Verification items for the finished model (mm, model axes). Face numbers are marked on the shaded views. Give positions to 0.01 mm unless a question says otherwise; leave off trailing zeros. Write each loop counter-clockwise with the first axis right and the second up, starting at its lowest first coordinate (ties: lowest second). Pieces come first, ordered by that corner, then holes. Notation, with made-up numbers: (63.5, 44) -> (115.5, 44) arc R17 ccw to (115.5, 76) -> close; hole circle Ø1 at (37, -13.5). An arc over 180 degrees is marked (long way). Use one line per item in the form item = value. Start each with the question number.
(1) Section check A-A, the plane x = 0. Record the cut outline in (y, z).
(2) Section check C-C, the plane z = 25.5. Record the cut outline in (x, y).
(3) Section check B-B, the plane y = 0. Record the cut outline in (x, z).
(4) Depth check by flat-ended pin: pin 1 Ø12 at (x, z) = (-1.5, 56) entering from -Y; pin 2 Ø6 at (y, z) = (-12, 59.5) entering from +X; pin 3 Ø2 at (x, y) = (1, -12.5) entering from +Z; pin 4 Ø5 at (y, z) = (16.5, 54) entering from +X. Enter the tip coordinate at first touch or a pass-through.
(5) Section check D-D, the plane y = -16.5. Record the cut outline in (x, z).
(6) Release check for a two-part mould opening along Y. For the marked faces 1, 2 and 3 record: pulls with the +Y half, pulls with the -Y half, needs draft (parallel to the pull), parting line crosses it, or undercut.
(7) Scan lines: L1, parallel to Y at x = 0, z = 79; L2, parallel to X at y = -5.5, z = 41; L3, parallel to X at y = -10.5, z = 83. Record each from-to range of solid material in increasing order.
from build123d import *

# Parameters (mm, degrees)
SKETCH1_R           = 22
SKETCH1_R_2         = 14.1
BOSS_EXTRUDE1_DEPTH = 100
CUT_EXTRUDE1_DEPTH  = 105.728219693


with BuildPart() as part:
    # Sketch1 → Boss-Extrude1 (new body)
    with BuildSketch(Plane.XY):
        Circle(SKETCH1_R)
        Circle(SKETCH1_R_2, mode=Mode.SUBTRACT)
    extrude(amount=BOSS_EXTRUDE1_DEPTH)

    # Sketch2 → Cut-Extrude1 (cut, through all)
    with BuildSketch(Plane(origin=(0, 0, 0), x_dir=(-1, 0, 0), z_dir=(0, 0, -1))):
        Polygon((0, 18.1), (4, 18.1), (4, 12.1), (-4, 12.1), (-4, 18.1), align=None)
    extrude(amount=-CUT_EXTRUDE1_DEPTH, mode=Mode.SUBTRACT)


solid = part.part
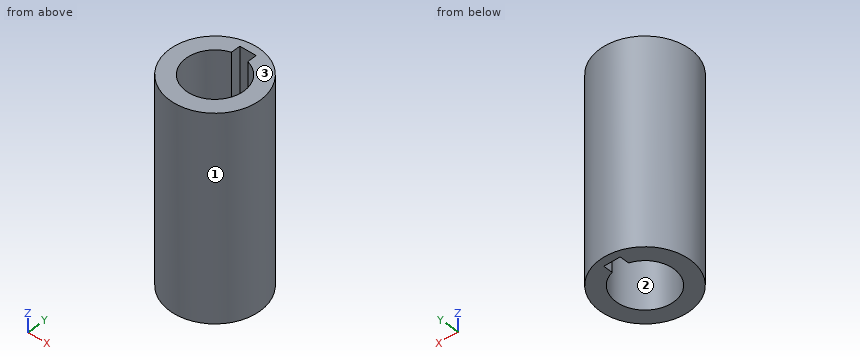
Completed:
q1.outline = (-22, 0) -> (-14.1, 0) -> (-14.1, 100) -> (-22, 100) -> close; (18.1, 0) -> (22, 0) -> (22, 100) -> (18.1, 100) -> close
q2.outline = circle Ø44 at (0, 0); hole (-4, 13.52) arc R14.1 ccw (long way) to (4, 13.52) -> (4, 18.1) -> (-4, 18.1) -> close
q3.outline = (-22, 0) -> (-14.1, 0) -> (-14.1, 100) -> (-22, 100) -> close; (14.1, 0) -> (22, 0) -> (22, 100) -> (14.1, 100) -> close
q4.pin_1 = -22
q4.pin_2 = 20.07
q4.pin_3 = through
q4.pin_4 = 16.97
q5.outline = (-14.55, 0) -> (14.55, 0) -> (14.55, 100) -> (-14.55, 100) -> close
q6.face_1 = parting line crosses it
q6.face_2 = undercut
q6.face_3 = needs draft
q7.L1 = -22 to -14.1, 18.1 to 22
q7.L2 = -21.3 to -12.98, 12.98 to 21.3
q7.L3 = -19.33 to -9.41, 9.41 to 19.33
